Here's how the part is built. I have some questions about the finished solid (model axes, mm). A direction names the side the tool comes from. Round coordinates to 2 decimals unless told otherwise and drop trailing zeros. Loops run counter-clockwise (first coordinate to the right, second up) from the corner with the lowest first, then second, coordinate; pieces in that order, holes last. Notation, with made-up numbers: M 25.25,47 L 58.25,47 A16 cw 58.25,70 Z; hole C 80,89.25 d4. An arc over 180 degrees is marked long. Use a Markdown table: item, result.
```python
from build123d import *

# Parameters (mm, degrees)
BOSS_EXTRUDE1_DEPTH = 20
SKETCH2_R           = 1.35
CUT_EXTRUDE2_DEPTH  = 12
SKETCH3_R           = 5
BOSS_EXTRUDE2_DEPTH = 17
SKETCH4_R           = 6
BOSS_EXTRUDE3_DEPTH = 7


with BuildPart() as part:
    # Sketch1 → Boss-Extrude1 (new body)
    with BuildSketch(Plane.XY):
        with BuildLine():
            Line((-5, -19.5), (3, -19.5))
            ThreePointArc((3, -19.5), (4.414213562, -18.914213562), (5, -17.5))
            Line((5, -17.5), (5, 17.5))
            ThreePointArc((5, 17.5), (4.414213562, 18.914213562), (3, 19.5))
            Line((3, 19.5), (-5, 19.5))
            Line((-5, 19.5), (-5, -19.5))
        make_face()
    extrude(amount=BOSS_EXTRUDE1_DEPTH)

    # Sketch2 → Cut-Extrude2 (cut)
    with BuildSketch(Plane.XY.offset(20)):
        with Locations((-0.5, 15.5)):
            Circle(SKETCH2_R)
        with Locations((-0.5, 5.5)):
            Circle(SKETCH2_R)
        with Locations((-0.5, -15.5)):
            Circle(SKETCH2_R)
        with Locations((-0.5, -5.5)):
            Circle(SKETCH2_R)
    extrude(amount=-CUT_EXTRUDE2_DEPTH, mode=Mode.SUBTRACT)

    # Sketch3 → Boss-Extrude2 (add)
    with BuildSketch(Plane(origin=(5, 0, 0), x_dir=(0, 0, -1), z_dir=(1, 0, 0))):
        with Locations((-10, 0)):
            Circle(SKETCH3_R)
    extrude(amount=BOSS_EXTRUDE2_DEPTH)

    # Sketch4 → Boss-Extrude3 (add)
    with BuildSketch(Plane(origin=(5, 0, 0), x_dir=(0, 0, -1), z_dir=(1, 0, 0))):
        with Locations((-10, 0)):
            Circle(SKETCH4_R)
    extrude(amount=BOSS_EXTRUDE3_DEPTH)


solid = part.part
```
Q1. For faces 1 (the cylindrical face through (8.451, 1.802, 4.277)), 2 (the cylindrical face through (0.226, -4.362, 14.084)), 3 (the flat face through (0, 0, 20)), which set-ups out of +Z, -Z, +X, -X, +Y, -Y let a thin tool reach every point of the face, with its end or its side?
Return value:
| item | result |
|---|---|
| face 1 | +X |
| face 2 | +Z |
| face 3 | +Z, +X, -X, +Y, -Y |
Q2. Will these pins go through, and if not, where does the flat tip stop? P1, Ø4, axis at x = 5, y = 7, coming from the -Z side; P2, Ø0.8, axis at x = -0.5, y = 15.5, coming from the +Z side; P3, Ø1.5, axis at y = 6.5, z = 2.5, coming from the +X side; P4, Ø6, axis at y = 8.5, z = 10, coming from the +X side.
Return value:
| item | result |
|---|---|
| P1 | stops at z = 0 |
| P2 | stops at z = 8 |
| P3 | stops at x = 5 |
| P4 | stops at x = 12 |
Q3. We'd pull the mould along Y, two halves only. Please class faces 4 (the flat face through (5, -4, 5)), 5 (the cylindrical face through (-0.676, -14.161, 14.084)), 6 (the flat face through (-1, 19.5, 10)), 7 (the flat face through (-1, 6, 8)): pulls with the +Y half, pulls with the -Y half, needs draft (parallel to the pull), parting line crosses it, or undercut.
Return value:
| item | result |
|---|---|
| face 4 | needs draft |
| face 5 | undercut |
| face 6 | pulls with the +Y half |
| face 7 | undercut |
Q4. Imagine slicing it at D-D, the plane z = 17.75. Please give me the cut outline in (x, y).
Return value:
| item | result |
|---|---|
| outline | M -5,-19.5 L 3,-19.5 A2 ccw 5,-17.5 L 5,17.5 A2 ccw 3,19.5 L -5,19.5 Z; hole C -0.5,-15.5 d2.7; hole C -0.5,-5.5 d2.7; hole C -0.5,5.5 d2.7; hole C -0.5,15.5 d2.7 |
Q5. Imagine slicing it at B-B, the plane x = -0.5. Please give me the cut outline in (y, z).
Return value:
| item | result |
|---|---|
| outline | M -19.5,0 L 19.5,0 L 19.5,20 L 16.85,20 L 16.85,8 L 14.15,8 L 14.15,20 L 6.85,20 L 6.85,8 L 4.15,8 L 4.15,20 L -4.15,20 L -4.15,8 L -6.85,8 L -6.85,20 L -14.15,20 L -14.15,8 L -16.85,8 L -16.85,20 L -19.5,20 Z |
Q6. Imagine slicing it at C-C, the plane y = 15.5. Please give me the cut outline in (x, z), then the cut area to 3 significant figures.
Return value:
| item | result |
|---|---|
| outline | M -5,0 L 5,0 L 5,20 L 0.85,20 L 0.85,8 L -1.85,8 L -1.85,20 L -5,20 Z |
| area | 168 mm^2 |
Q7. Imagine slicing it at A-A, the plane z = 10. Please give me the cut outline in (x, y).
Return value:
| item | result |
|---|---|
| outline | M -5,-19.5 L 3,-19.5 A2 ccw 5,-17.5 L 5,-6 L 12,-6 L 12,-5 L 22,-5 L 22,5 L 12,5 L 12,6 L 5,6 L 5,17.5 A2 ccw 3,19.5 L -5,19.5 Z; hole C -0.5,-15.5 d2.7; hole C -0.5,-5.5 d2.7; hole C -0.5,5.5 d2.7; hole C -0.5,15.5 d2.7 |
Q8. I need wall thicknesses on line 1 (Y direction, x = -0.5, z = 10.5); line 2 (Y direction, x = 0.25, z = 9); line 3 (X direction, y = -9, z = 15). Which ranges of each line are inside material? Lowest first, please. Write a range as from..to.
Return value:
| item | result |
|---|---|
| line 1 | y = -19.5..-16.85, -14.15..-6.85, -4.15..4.15, 6.85..14.15, 16.85..19.5 |
| line 2 | y = -19.5..-16.62, -14.38..-6.62, -4.38..4.38, 6.62..14.38, 16.62..19.5 |
| line 3 | x = -5..5 |
